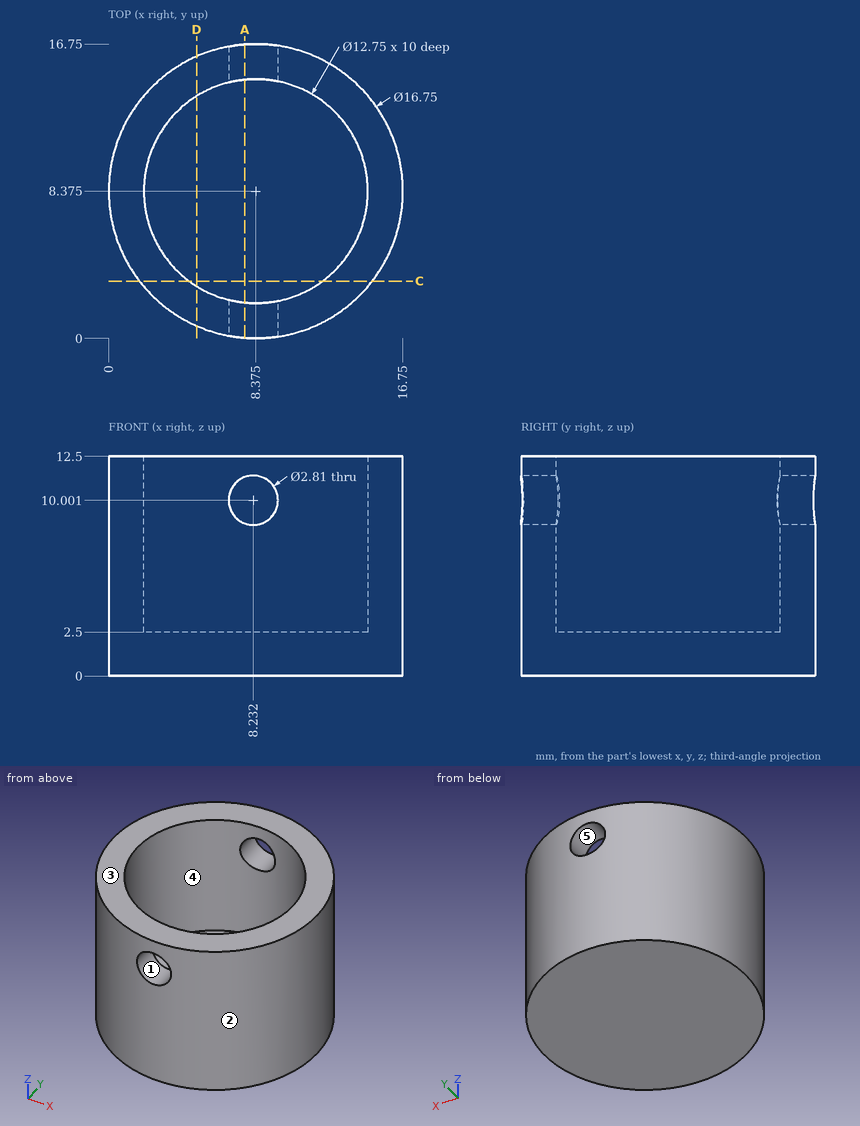
Print and shaded views of the part. All mm, measured from the part's lowest x, y and z. A direction names the side the tool comes from. Coordinates: 2 decimals unless noted, no trailing zeros. Loops run counter-clockwise (first coordinate to the right, second up) from the corner with the lowest first, then second, coordinate; pieces in that order, holes last. Notation, with made-up numbers: (57.25, -22) -> (113.25, -22) arc R12 cw to (113.25, -17) -> close; hole circle Ø10 at (66.5, 26.25). An arc over 180 degrees is marked (long way). Use one line per item in the form item = value. Start each with the question number.
(1) Cut at C-C on y = 3.25. Give the cut face in (x, z).
(2) Flat gauge pins, fed straight in: pin 1 (5 mm diameter, centred on y = 3.5, z = 8, fed in from +X); pin 2 (1 mm diameter, centred on y = 2, z = 1.5, fed in from +X) (1 decimal); pin 3 (1.5 mm diameter, centred on x = 6.5, z = 4.5, fed in from +Y). Where does each tip first touch, or does it go through?
(3) Cut at A-A on x = 7.75. Give the cut face in (y, z).
(4) Tool access for the marked faces 4 and 5: list every direction of +Z, -Z, +X, -X, +Y, -Y with a clear straight run to the whole face (end or side of a thin tool).
(5) Cut at D-D on x = 5. Give the cut face in (y, z).
(6) Probe probe 1 along Z at (x, y) = (7.5, 9.5); probe 2 along X at (y, z) = (7.75, 11); probe 3 along X at (y, z) = (11.75, 3.5) (1 decimal). List the from-to ranges inside material, lowest first. Write a range as from..to.
(7) Pull direction X, two halves, no side cores. Call the marked faces 1, 2 and 3: pulls with the +X half, pulls with the -X half, needs draft (parallel to the pull), parting line crosses it, or undercut.
Values:
q1.outline = (1.75, 0) -> (15, 0) -> (15, 12.5) -> (12.17, 12.5) -> (12.17, 2.5) -> (4.58, 2.5) -> (4.58, 12.5) -> (1.75, 12.5) -> close
q2.pin_1 = 16.41
q2.pin_2 = 14.3
q2.pin_3 = 16.67
q3.outline = (0.02, 0) -> (16.73, 0) -> (16.73, 8.68) -> (14.72, 8.68) -> (14.72, 2.5) -> (2.03, 2.5) -> (2.03, 8.68) -> (0.02, 8.68) -> close; (0.02, 11.32) -> (2.03, 11.32) -> (2.03, 12.5) -> (0.02, 12.5) -> close; (14.72, 11.32) -> (16.73, 11.32) -> (16.73, 12.5) -> (14.72, 12.5) -> close
q4.face_4 = +Z
q4.face_5 = +Y, -Y
q5.outline = (0.71, 0) -> (16.04, 0) -> (16.04, 12.5) -> (13.78, 12.5) -> (13.78, 2.5) -> (2.97, 2.5) -> (2.97, 12.5) -> (0.71, 12.5) -> close
q6.probe_1 = 0..2.5
q6.probe_2 = 0.02..2.03, 14.72..16.73
q6.probe_3 = 0.7..3, 13.8..16
q7.face_1 = undercut
q7.face_2 = parting line crosses it
q7.face_3 = needs draft
